Verification items for the finished model (mm, model axes). A direction names the side the tool comes from. Coordinates: 2 decimals unless noted, no trailing zeros. Order: outer loops, then holes, each group sorted by start corner. A loop starts at its lowest first (then second) coordinate and runs counter-clockwise, first axis right, second up. Notation, with made-up numbers: M 18.5,-28 L 41.5,-28 A27 ccw 41.5,-6 Z; hole C 11.5,78.5 d4. An arc over 180 degrees is marked long. Return JSON: item names as keys, results as strings.
Autodesk Inventor part; units mm, degrees
ref_plane "YZ Plane" through (0, 0, 0) normal (1, 0, 0) x (0, 1, 0)
ref_plane "XZ Plane" through (0, 0, 0) normal (0, 1, 0) x (-1, 0, 0)
ref_plane "XY Plane" through (0, 0, 0) normal (0, 0, 1) x (1, 0, 0)
sketch "Sketch1" plane through (0, 0, 0) normal (0, 1, 0) x (-1, 0, 0)
  arc A0 (-15, 0) -> (0, -15) centre (0, 0) ccw
  arc A1 (3.5986, 8.9) -> (3.5986, -8.9) centre (0, 0) ccw
  line L0 (24.0501, -8.9) -> (3.5986, -8.9)
  line L1 (0, -15) -> (9.6509, -15)
  arc A2 (9.6509, -15) -> (16.5791, -15) centre (13.115, -13) ccw
  circle A3 centre (13.115, 13.6) radius 1.5
  arc A4 (25.389, 3.3975) -> (24.0501, 4.7088) centre (20.7501, 0) ccw
  arc A5 (25.389, -3.3975) -> (25.389, 3.3975) centre (26.23, 0) ccw
  arc A6 (24.0501, -4.7088) -> (25.389, -3.3975) centre (20.7501, 0) ccw
  line L2 (24.0501, -4.7088) -> (24.0501, -8.9)
  line L3 (24.0501, -8.9) -> (3.5986, -8.9)
  arc A7 (3.5986, 8.9) -> (3.5986, -8.9) centre (0, 0) ccw
  line L4 (3.5986, 8.9) -> (24.0501, 8.9)
  line L5 (24.0501, 8.9) -> (24.0501, 4.7088)
  circle A8 centre (13.115, -13) radius 1.5
  line L6 (0, -15) -> (9.6509, -15)
  arc A9 (9.6509, -15) -> (16.5791, -15) centre (13.115, -13) ccw
  line L7 (16.5791, -15) -> (41.23, -15)
  line L8 (41.23, -15) -> (41.23, 18.9874)
  line L9 (41.23, 18.9874) -> (-15, 18.9874)
  line L10 (-15, 18.9874) -> (-15, 0)
  arc A10 (-15, 0) -> (0, -15) centre (0, 0) ccw
  line L11 (16.5791, -15) -> (41.23, -15)
extrude "Extrusion1" add sketch "Sketch1" along normal blind 2
fillet "Fillet1" radius 15 1 edges at (-41.23, 1, -15)
properties part number "Dock top2 V2" material "Acrylic"
Q1. Material ranges on line 1 along Z through (x, y) = (0, 0.5); line 2 along Z through (x, y) = (-19, 0.55); line 3 along X through (y, z) = (0.6, 0), recorded low to high.
Values:
{"line 1": "-15 to -9.6, 9.6 to 18.99", "line 2": "-15 to -8.9, 8.9 to 18.99", "line 3": "-41.23 to -29.73, 9.6 to 15"}
Q2. Cross-section at C-C, the plane y = 0.3. Record the boundary of the cut face in (x, z) (1 decimal), and give its area (3 significant figures).
Values:
{"outline": "M -41.2,0 A15 ccw -26.2,-15 L -16.6,-15 A4 ccw -9.7,-15 L 0,-15 A15 ccw 15,0 L 15,19 L -41.2,19 Z; hole M -25.4,-3.4 A5.7 ccw -24.1,-4.7 L -24.1,-8.9 L -3.6,-8.9 A9.6 ccw long -3.6,8.9 L -24.1,8.9 L -24.1,4.7 A5.8 ccw -25.4,3.4 A3.5 ccw long Z; hole C -13.1,-13 d3; hole C -13.1,13.6 d3", "area": "1,200 mm^2"}
Q3. Go/stop test with flat-tipped pins: pin 1 (2.5 mm diameter, centred on x = -13.115, z = -13, fed in from +Y); pin 2 (2 mm diameter, centred on x = -20.5, z = -10.5, fed in from -Y); pin 3 (1 mm diameter, centred on y = 1, z = -6, fed in from +X). Record where each tip stops, or that it passes through.
Values:
{"pin 1": "through", "pin 2": "y = 0", "pin 3": "x = 13.96"}
Q4. Cross-section at B-B, the plane x = -20. Record the boundary of the cut face in (y, z).
Values:
{"outline": "M 0,-15 L 2,-15 L 2,-8.9 L 0,-8.9 Z; M 0,8.9 L 2,8.9 L 2,18.99 L 0,18.99 Z"}
Q5. Draft check along X on faces 1 (the face through (-14, 1, 8.9)), 2 (the face through (-21, 1, -15)), 3 (the face through (-24.78, 0.99, -4.1)), 4 (the face through (15, 1, 10)). Enter one of: pulls with the +X half, pulls with the -X half, needs draft (parallel to the pull), parting line crosses it, or undercut.
Values:
{"face 1": "undercut", "face 2": "needs draft", "face 3": "undercut", "face 4": "pulls with the +X half"}
Q6. Cross-section at A-A, the plane z = 13.6. Record the boundary of the cut face in (x, y) (3 decimals).
Values:
{"outline": "M -41.23,0 L -14.615,0 L -14.615,2 L -41.23,2 Z; M -11.615,0 L 15,0 L 15,2 L -11.615,2 Z"}
Q7. Tool access check on faces 5 (the face through (-5, 1, -15)), 6 (the face through (-41.23, 1, 9)), 7 (the face through (-24.76, 0.99, 4.12)). Record the directions out of +Z, -Z, +X, -X, +Y, -Y that give a thin tool (end or side, any length) a straight path to the whole face; none if there is none.
Values:
{"face 5": "-Z, +X, +Y, -Y", "face 6": "+Z, -Z, -X, +Y, -Y", "face 7": "+Y, -Y"}
Q8. Cross-section at D-D, the plane x = -33.5. Record the boundary of the cut face in (y, z).
Values:
{"outline": "M 0,-13.12 L 2,-13.12 L 2,18.99 L 0,18.99 Z"}
